```python
from build123d import *

# Parameters (mm, degrees)
F0_R     = 10
F1_DEPTH = 20
F2_DEPTH = 50
F3_SIZE  = 2


with BuildPart() as f1:
    # F0 (on Front) → F1 (new body)
    with BuildSketch(Plane.XZ):
        with BuildLine():
            ThreePointArc((2.083333, -24.913043), (18.399502, -16.92508), (25, 0))
            ThreePointArc((25, 0), (18.399502, 16.92508), (2.083333, 24.913043))
            ThreePointArc((2.083333, 24.913043), (-25, 0), (2.083333, -24.913043))
        make_face()
        Circle(F0_R, mode=Mode.SUBTRACT)
        with BuildLine():
            ThreePointArc((2.083333, 24.913043), (18.399502, 16.92508), (25, 0))
            ThreePointArc((25, 0), (18.399502, -16.92508), (2.083333, -24.913043))
            Line((2.083333, -24.913043), (91.458333, -17.43913))
            ThreePointArc((91.458333, -17.43913), (72.5, 0), (91.458333, 17.43913))
            Line((91.458333, 17.43913), (2.083333, 24.913043))
        make_face()
        with BuildLine():
            ThreePointArc((107.5, 0), (102.879651, 11.847556), (91.458333, 17.43913))
            ThreePointArc((91.458333, 17.43913), (72.5, 0), (91.458333, -17.43913))
            ThreePointArc((91.458333, -17.43913), (102.879651, -11.847556), (107.5, 0))
        make_face()
        with Locations((90, 0)):
            Circle(F0_R, mode=Mode.SUBTRACT)
    extrude(amount=F1_DEPTH)

    # F0 (on Front) → F2 (join)
    with BuildSketch(Plane.XZ):
        with BuildLine():
            ThreePointArc((2.083333, -24.913043), (18.399502, -16.92508), (25, 0))
            ThreePointArc((25, 0), (18.399502, 16.92508), (2.083333, 24.913043))
            ThreePointArc((2.083333, 24.913043), (-25, 0), (2.083333, -24.913043))
        make_face()
        Circle(F0_R, mode=Mode.SUBTRACT)
    extrude(amount=F2_DEPTH)

    # F3
    f3_edges = [f1.edges().sort_by_distance(p)[0] for p in [
        (-10, 0, 0),
        (10, -25, 0),
        (-10, -50, 0),
        (-2.083333, -50, 24.913043),
        (80, -20, 0),
    ]]
    chamfer(f3_edges, length=F3_SIZE)


solid = f1.part
```
Work out the finished part from the listing and answer in its coordinate system (mm). Round coordinates to 2 decimals unless told otherwise and drop trailing zeros. Write each loop counter-clockwise with the first axis right and the second up, starting at its lowest first coordinate (ties: lowest second). Pieces come first, ordered by that corner, then holes. Notation, with made-up numbers: (4.5, 30.5) - (53.5, 30.5) arc R24 ccw to (53.5, 53.5) - close; hole circle Ø10 at (28.5, 73.25). An arc over 180 degrees is marked (long way). Return JSON: item names as keys, results as strings. Group by question number.
Q1. Each of these flat-tipped pins is pushed along its axis until it touches: pin 1 Ø12 at (x, z) = (32, 9) entering from +Y; pin 2 Ø10 at (x, y) = (-6.5, -39) entering from -Z; pin 3 Ø10 at (y, z) = (-24, -12) entering from -X; pin 4 Ø6 at (x, y) = (56, -13.5) entering from -Z. Where does it stop, or does it pass through?
Q2. The part is cut by section D-D on z = 5.5. Count the separate pieces of the cut face and the enclosed holes in it, then the cut area to 3 significant figures.
Q3. The mould has two halves that part along X. Classify faces 1 (the flat face through (46.15, -9.86, -21.23)), 2 (the flat face through (10, -50, -10)), 3 (the cylindrical face through (-2.17, -24.68, -9.76)): released by +X, released by -X, zero draft, split by the parting line, or undercut.
Q4. The part is cut by section C-C on y = -28. Write down the section's boundary in (x, z), then the cut area to 3 significant figures.
Q5. The part is cut by section A-A on x = 0. Write down the section's boundary in (y, z), then the cut area to 3 significant figures.
Q6. Find the intervals of material crossed by L1, parallel to Z at x = 0, y = -14.5; L2, parallel to X at y = -11, z = -9; L3, parallel to Y at x = 37, z = -19.5, in increasing order.
Q7. The part is cut by section B-B on y = -9.5. Write down the section's boundary in (x, z).
Solved:
{
 "1": {"pin 1": "y = 0", "pin 2": "z = -24.95", "pin 3": "x = -24", "pin 4": "z = -20.66"},
 "2": {"separate pieces": "3", "enclosed holes": "0", "area": "2,900 mm²"},
 "3": {"face 1": "released by +X", "face 2": "zero draft", "face 3": "undercut"},
 "4": {"outline": "(2.08, -24.91) arc R25 ccw to (25, 0) arc R25 ccw to (2.08, 24.91) arc R25 ccw (long way) to start; hole circle Ø20 at (0, 0)", "area": "1,650 mm²"},
 "5": {"outline": "(-50, -23) - (-48, -25) - (0, -25) - (0, -12) - (-2, -10) - (-48, -10) - (-50, -12) - close; (-50, 12) - (-48, 10) - (-2, 10) - (0, 12) - (0, 25) - (-48, 25) - (-50, 23) - close", "area": "1,490 mm²"},
 "6": {"L1": "-25 to -10, 10 to 25", "L2": "-23.32 to -4.36, 4.36 to 85.64, 94.36 to 105.01", "L3": "-20 to 0"},
 "7": {"outline": "(2.08, -24.91) - (91.46, -17.44) arc R17.5 ccw to (91.46, 17.44) - (2.08, 24.91) arc R25 ccw (long way) to start; hole circle Ø20 at (0, 0); hole circle Ø20 at (90, 0)"}
}
